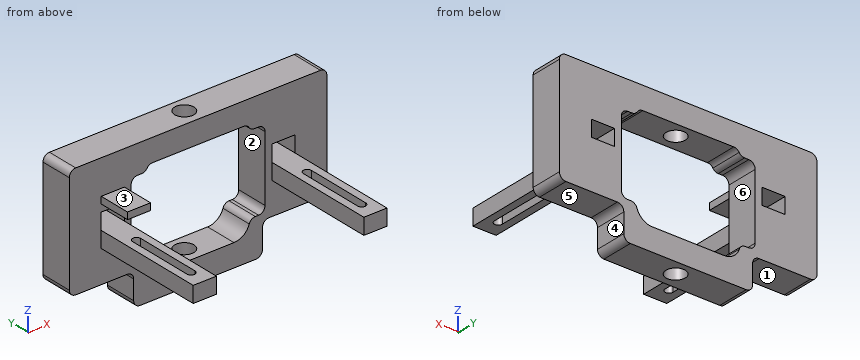
```python
from build123d import *

# Parameters (mm, degrees)
SKETCH_1_W          = 80
SKETCH_1_H          = 35
EXTRUDE_1_DEPTH     = 10
SKETCH_2_W          = 7.2
SKETCH_2_H          = 5
SKETCH_2_H_2        = 5.001973484
CUT_EXTRUDE_1_DEPTH = 20
SKETCH_6_W          = 7.19
SKETCH_6_H          = 5
EXTRUDE_7_DEPTH     = 45
SKETCH_7_R          = 1.25
CUT_EXTRUDE_2_DEPTH = 30
SKETCH_8_W          = 40
SKETCH_8_H          = 10
EXTRUDE_8_DEPTH     = 10
SKETCH_10_W         = 32.274232457
SKETCH_10_H         = 31.000986742
CUT_EXTRUDE_3_DEPTH = 10
FILLET_1_R          = 5
FILLET_2_R          = 2
SKETCH_11_R         = 3
CUT_EXTRUDE_4_DEPTH = 50
CUT_EXTRUDE_5_DEPTH = 50
FILLET_3_R          = 2
SKETCH_13_W         = 7.18
SKETCH_13_H         = 2.109830921
EXTRUDE_9_DEPTH     = 10
SKETCH_14_W         = 41.600257034
SKETCH_14_H         = 24.338135392
CUT_EXTRUDE_6_DEPTH = 10
FILLET_5_R          = 2


with BuildPart() as part:
    # 草图1 → 凸台-拉伸1 (new body)
    with BuildSketch(Plane(origin=(0, 0, 0), x_dir=(1, 0, 0), z_dir=(0, 1, 0))):
        with Locations((21.527777778, -7.5)):
            Rectangle(SKETCH_1_W, SKETCH_1_H)
    extrude(amount=EXTRUDE_1_DEPTH)

    # 草图2 → 切除-拉伸1 (cut)
    with BuildSketch(Plane(origin=(0, 10, 0), x_dir=(1, 0, 0), z_dir=(0, 1, 0))):
        with Locations((-4.972222222, -7.500493371)):
            Rectangle(SKETCH_2_W, SKETCH_2_H)
        with Locations((48.027777778, -7.499506629)):
            Rectangle(SKETCH_2_W, SKETCH_2_H_2)
    extrude(amount=-CUT_EXTRUDE_1_DEPTH, mode=Mode.SUBTRACT)

    # 草图6 → 凸台-拉伸7 (add)
    with BuildSketch(Plane(origin=(0, 10, 0), x_dir=(1, 0, 0), z_dir=(0, 1, 0))):
        with Locations((-4.977222222, -2.500493371)):
            Rectangle(SKETCH_6_W, SKETCH_6_H)
        with Locations((48.032777778, -2.500493371)):
            Rectangle(SKETCH_6_W, SKETCH_6_H)
    extrude(amount=-EXTRUDE_7_DEPTH)

    # 草图7 → 切除-拉伸2 (cut)
    with BuildSketch(Plane.XY.offset(5.000493371)):
        with Locations((-4.972222222, -12)):
            Circle(SKETCH_7_R)
        with Locations((48.027777778, -12)):
            Circle(SKETCH_7_R)
    extrude(amount=-CUT_EXTRUDE_2_DEPTH, mode=Mode.SUBTRACT)

    # 草图8 → 凸台-拉伸8 (add)
    with BuildSketch(Plane(origin=(0, 0, -10), x_dir=(-1, 0, 0), z_dir=(0, 0, -1))):
        with Locations((-21.527777778, 5)):
            Rectangle(SKETCH_8_W, SKETCH_8_H)
    extrude(amount=EXTRUDE_8_DEPTH)

    # 草图10 → 切除-拉伸3 (cut)
    with BuildSketch(Plane(origin=(0, 10, 0), x_dir=(1, 0, 0), z_dir=(0, 1, 0))):
        with Locations((21.527777778, -2.5)):
            Rectangle(SKETCH_10_W, SKETCH_10_H)
    extrude(amount=-CUT_EXTRUDE_3_DEPTH, mode=Mode.SUBTRACT)

    # 圆角1
    fillet_1_edges = [part.edges().sort_by_distance(p)[0] for p in [
        (37.664894006, 5, -13.000493371),
        (5.390661549, 5, -13.000493371),
    ]]
    fillet(fillet_1_edges, radius=FILLET_1_R)

    # 圆角2
    fillet_2_edges = [part.edges().sort_by_distance(p)[0] for p in [
        (37.664894006, 5, 18.000493371),
        (5.390661549, 5, 18.000493371),
    ]]
    fillet(fillet_2_edges, radius=FILLET_2_R)

    # 草图11 → 切除-拉伸4 (cut)
    with BuildSketch(Plane.XY.offset(25)):
        with Locations(Location((21.527777778, 5.231122454, 0), (0, 0, 180))):
            Circle(SKETCH_11_R)
    extrude(amount=-CUT_EXTRUDE_4_DEPTH, mode=Mode.SUBTRACT)

    # 草图12 → 切除-拉伸5 (cut)
    with BuildSketch(Plane.XY.offset(5.000493371)):
        with BuildLine():
            Line((-3.722222222, -9.086156221), (-3.722222222, -29.777694538))
            ThreePointArc((-3.722222222, -29.777694538), (-4.972222222, -31.027694538), (-6.222222222, -29.777694538))
            Line((-6.222222222, -29.777694538), (-6.222222222, -9.086156221))
            ThreePointArc((-6.222222222, -9.086156221), (-4.972222222, -7.836156221), (-3.722222222, -9.086156221))
        make_face()
        with BuildLine():
            Line((46.777777778, -9.086156221), (46.777777778, -29.777694538))
            ThreePointArc((46.777777778, -29.777694538), (48.027777778, -31.027694538), (49.277777778, -29.777694538))
            Line((49.277777778, -29.777694538), (49.277777778, -9.086156221))
            ThreePointArc((49.277777778, -9.086156221), (48.027777778, -7.836156221), (46.777777778, -9.086156221))
        make_face()
    extrude(amount=-CUT_EXTRUDE_5_DEPTH, mode=Mode.SUBTRACT)

    # 圆角3
    fillet_3_edges = [part.edges().sort_by_distance(p)[0] for p in [
        (41.527777778, 5, -10),
        (1.527777778, 5, -10),
        (41.527777778, 5, -20),
        (1.527777778, 5, -20),
        (61.527777778, 5, 25),
        (-18.472222222, 5, 25),
        (-18.472222222, 5, -10),
        (61.527777778, 5, -10),
    ]]
    fillet(fillet_3_edges, radius=FILLET_3_R)

    # 草图13 → 凸台-拉伸9 (add)
    with BuildSketch(Plane.XZ):
        with Locations((-4.972222222, 13.322503868)):
            Rectangle(SKETCH_13_W, SKETCH_13_H)
    extrude(amount=EXTRUDE_9_DEPTH)

    # 草图14 → 切除-拉伸6 (cut)
    with BuildSketch(Plane(origin=(0, 10, 0), x_dir=(1, 0, 0), z_dir=(0, 1, 0))):
        with Locations((21.527777778, -4)):
            Rectangle(SKETCH_14_W, SKETCH_14_H)
    extrude(amount=-CUT_EXTRUDE_6_DEPTH, mode=Mode.SUBTRACT)

    # 圆角5
    fillet_5_edges = [part.edges().sort_by_distance(p)[0] for p in [
        (5.397778538, 5, 16.169067696),
        (5.393504088, 5, -8.169067696),
        (37.662051468, 5, -8.169067696),
        (0.727649261, 5, -8.169067696),
        (37.657777017, 5, 16.169067696),
        (42.327906295, 5, 16.169067696),
        (0.727649261, 5, 16.169067696),
        (42.327906295, 5, -8.169067696),
    ]]
    fillet(fillet_5_edges, radius=FILLET_5_R)


solid = part.part
```
Part model, mm, in its own coordinate system. Face numbers are marked on the shaded views. A direction names the side the tool comes from. Round coordinates to 2 decimals unless told otherwise and drop trailing zeros. Order: outer loops, then holes, each group sorted by start corner. A loop starts at its lowest first (then second) coordinate and runs counter-clockwise, first axis right, second up. Notation, with made-up numbers: M 16,89 L 58,89 A12 ccw 58,107 Z; hole C -5.75,31 d1. An arc over 180 degrees is marked long. Put each result on its own line as item: value. Start each with the question number.
1. Slice it at C-C on x = 23. List the corners of the cut face in (y, z), then the cut area to 3 significant figures.
2. Two-plate mould, pull along X, no slides. Class the marked faces 4, 5 and 6: +X half, -X half, draft (parallel to the pull), parting line (faces both ways), or undercut.
3. Drill centre lines: probe 1 along Z at (x, y) = (22, 2); probe 2 along Y at (x, z) = (47.5, 16); probe 3 along Z at (x, y) = (-6, 8). Where is each one in solid material? Low to high. Write a range as [from, to].
4. Drop flat-ended pins along their axis: pin 1 (2 mm diameter, centred on x = -5.5, y = -7, fed in from -Z); pin 2 (5.5 mm diameter, centred on y = -18.5, z = 2.5, fed in from +X); pin 3 (1.1 mm diameter, centred on y = -5, z = 13.5, fed in from +X); pin 4 (1.5 mm diameter, centred on x = -10, y = -26, fed in from -Z). Give the stop position or say it passes through.
5. Slice it at A-A on z = 6. List the corners of the cut face in (x, y), then the cut area to 3 significant figures.
6. Slice it at D-D on z = 20. List the corners of the cut face in (x, y), then the cut area to 3 significant figures.
7. Tool access for the marked faces 1, 2 and 3: list every direction of +Z, -Z, +X, -X, +Y, -Y with a clear straight run to the whole face (end or side of a thin tool).
8. Slice it at B-B on y = -5.5. List the corners of the cut face in (x, z), then the cut area to 3 significant figures.
Findings:
1. outline: M 0,-20 L 2.62,-20 L 2.62,-13 L 0,-13 Z; M 0,18 L 2.62,18 L 2.62,25 L 0,25 Z; M 7.85,-20 L 10,-20 L 10,-13 L 7.85,-13 Z; M 7.85,18 L 10,18 L 10,25 L 7.85,25 Z
1. area: 66.8 mm2
2. face 4: +X half
2. face 5: draft
2. face 6: undercut
3. probe 1: [-20, -13], [18, 25]
3. probe 2: [0, 10]
3. probe 3: [-10, 5], [10, 25]
4. pin 1: z = 0
4. pin 2: x = 51.63
4. pin 3: x = -1.38
4. pin 4: through
5. outline: M -18.47,0 L -8.57,0 L -8.57,10 L -18.47,10 Z; M -1.37,0 L 0.73,0 L 0.73,10 L -1.37,10 Z; M 42.33,0 L 44.43,0 L 44.43,10 L 42.33,10 Z; M 51.63,0 L 61.53,0 L 61.53,10 L 51.63,10 Z
5. area: 240 mm2
6. outline: M -18.47,0 L 61.53,0 L 61.53,10 L -18.47,10 Z; hole C 21.53,5.23 d6
6. area: 772 mm2
7. face 1: -Z, -X, +Y, -Y
7. face 2: +Y, -Y
7. face 3: +Z, +X, -X, -Y
8. outline: M -8.57,0 L -1.38,0 L -1.38,5 L -8.57,5 Z; M -8.56,12.27 L -1.38,12.27 L -1.38,14.38 L -8.56,14.38 Z; M 44.44,0 L 51.63,0 L 51.63,5 L 44.44,5 Z
8. area: 87.0 mm2
